Verification items for this drawing (mm, ordinates from the low corner). Round coordinates to 2 decimals unless told otherwise and drop trailing zeros. Order: outer loops, then holes, each group sorted by start corner. A loop starts at its lowest first (then second) coordinate and runs counter-clockwise, first axis right, second up. Notation, with made-up numbers: (-20, 44) -> (-6, 44) arc R38 ccw to (-6, 82) -> close; hole circle Ø5 at (77.5, 40). An arc over 180 degrees is marked (long way). Return JSON: item names as keys, results as strings. Group by question number.
Item 1: Sectioned sample at A-A on y = 3.45. Record the cut outline in (x, z), plus the area to 3 significant figures.
Item 2: Draft check along X on the marked faces 1, 2 and 3. Enter one of: pulls with the +X half, pulls with the -X half, needs draft (parallel to the pull), parting line crosses it, or undercut.
Item 3: Scan lines: probe 1 along X at (y, z) = (1.35, 60.2); probe 2 along X at (y, z) = (1.55, 62.5); probe 3 along Z at (x, y) = (18, 4.15). Record each from-to range of solid material in increasing order. Write a range as from..to.
Item 4: Sectioned sample at C-C on x = 39. Record the cut outline in (y, z), plus the area to 3 significant figures.
Item 5: Sectioned sample at B-B on z = 62.5. Record the cut outline in (x, y), plus the area to 3 significant figures.
Item 6: Sectioned sample at D-D on z = 13. Record the cut outline in (x, y), plus the area to 3 significant figures.
Item 7: Depth check by flat-ended pin: pin 1 Ø1 at (y, z) = (2.5, 22.5) entering from +X; pin 2 Ø1 at (x, y) = (16.5, 2.5) entering from -Z; pin 3 Ø2 at (x, y) = (30.5, 2) entering from -Z. Enter the tip coordinate at first touch or a pass-through.
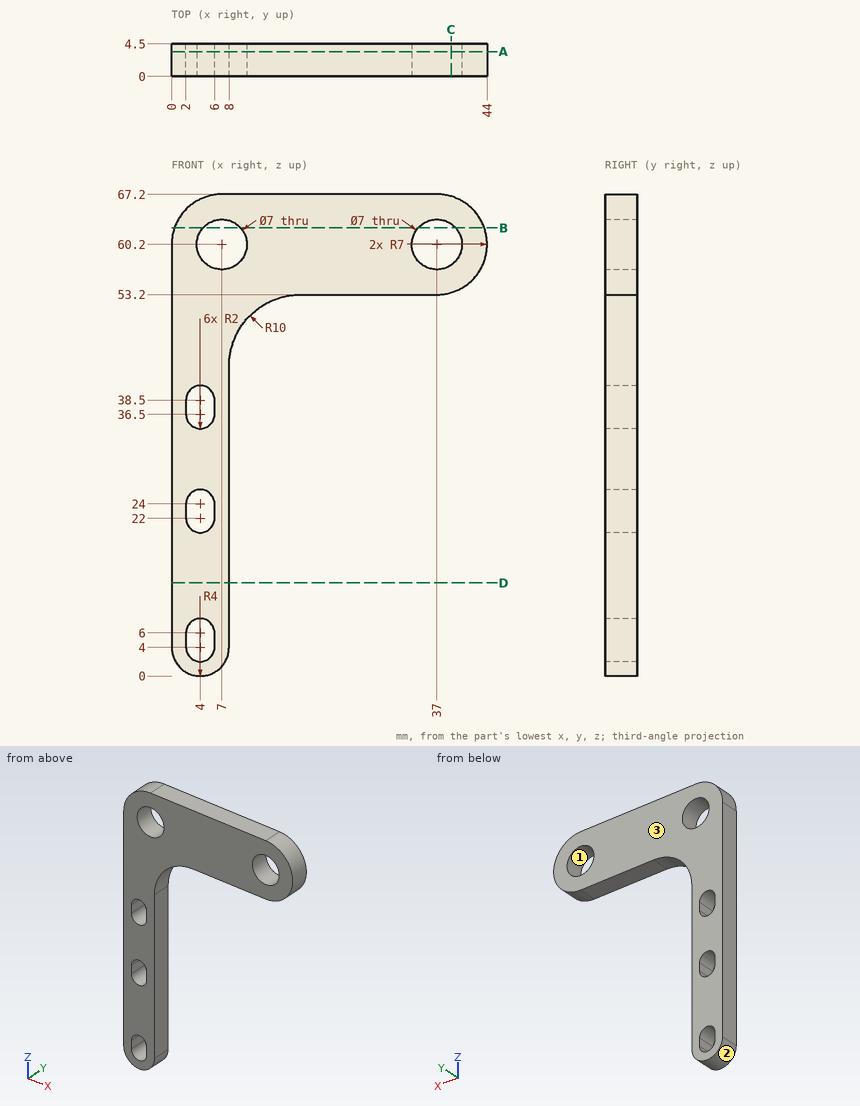
Recorded:
{
 "1": {"outline": "(0, 4) arc R4 ccw to (8, 4) -> (8, 43.2) arc R10 cw to (18, 53.2) -> (37, 53.2) arc R7 ccw to (37, 67.2) -> (7, 67.2) arc R7 ccw to (0, 60.2) -> close; hole (2, 4) arc R2 ccw to (6, 4) -> (6, 6) arc R2 ccw to (2, 6) -> close; hole (2, 22) arc R2 ccw to (6, 22) -> (6, 24) arc R2 ccw to (2, 24) -> close; hole (2, 36.5) arc R2 ccw to (6, 36.5) -> (6, 38.5) arc R2 ccw to (2, 38.5) -> close; hole circle Ø7 at (7, 60.2); hole circle Ø7 at (37, 60.2)", "area": "886 mm²"},
 "2": {"face 1": "undercut", "face 2": "parting line crosses it", "face 3": "needs draft"},
 "3": {"probe 1": "0..3.5, 10.5..33.5, 40.5..44", "probe 2": "0.39..4.36, 9.64..34.36, 39.64..43.61", "probe 3": "53.2..67.2"},
 "4": {"outline": "(0, 53.49) -> (4.5, 53.49) -> (4.5, 57.33) -> (0, 57.33) -> close; (0, 63.07) -> (4.5, 63.07) -> (4.5, 66.91) -> (0, 66.91) -> close", "area": "34.5 mm²"},
 "5": {"outline": "(0.39, 0) -> (4.36, 0) -> (4.36, 4.5) -> (0.39, 4.5) -> close; (9.64, 0) -> (34.36, 0) -> (34.36, 4.5) -> (9.64, 4.5) -> close; (39.64, 0) -> (43.61, 0) -> (43.61, 4.5) -> (39.64, 4.5) -> close", "area": "147 mm²"},
 "6": {"outline": "(0, 0) -> (8, 0) -> (8, 4.5) -> (0, 4.5) -> close", "area": "36.0 mm²"},
 "7": {"pin 1": "x = 8", "pin 2": "z = 53", "pin 3": "z = 53.2"}
}
